Geometry: final body of the model. Coordinates: model frame, mm. A direction names the side the tool comes from. Coordinates: 2 decimals unless noted, no trailing zeros. Loops run counter-clockwise (first coordinate to the right, second up) from the corner with the lowest first, then second, coordinate; pieces in that order, holes last. Notation, with made-up numbers: (39.5, 24.5) - (72.5, 24.5) arc R24 ccw to (72.5, 51.5) - close; hole circle Ø1 at (53, -32.5). An arc over 180 degrees is marked (long way). Return JSON: item names as keys, results as strings.
from build123d import *

# Parameters (mm, degrees)
SKETCH1_R           = 4
SKETCH1_R_2         = 6
SKETCH1_R_3         = 9
BOSS_EXTRUDE1_DEPTH = 8
SKETCH2_R           = 4
BOSS_EXTRUDE2_DEPTH = 3
SKETCH3_R           = 6
BOSS_EXTRUDE3_DEPTH = 3


with BuildPart() as part:
    # Sketch1 → Boss-Extrude1 (new body)
    with BuildSketch(Plane(origin=(0, 0, 0), x_dir=(1, 0, 0), z_dir=(0, 1, 0))):
        with BuildLine():
            Line((82, 0), (0, 0))
            Line((0, 0), (-45.003147253, 18.182451735))
            ThreePointArc((-45.003147253, 18.182451735), (-54.304086029, 15.690272701), (-54.472135955, 6.06269888))
            Line((-54.472135955, 6.06269888), (-18.061799059, -44.051830542))
            ThreePointArc((-18.061799059, -44.051830542), (-9.061799059, -50.590713294), (2.062812738, -50.590713294))
            Line((2.062812738, -50.590713294), (85.708203932, -23.412678196))
            ThreePointArc((85.708203932, -23.412678196), (93.852260087, -10.12278642), (82, 0))
        make_face()
        with Locations(Location((-48, 10.764980899, 0), (0, 0, 270))):
            Circle(SKETCH1_R, mode=Mode.SUBTRACT)
        with Locations(Location((82, -12, 0), (0, 0, 270))):
            Circle(SKETCH1_R_2, mode=Mode.SUBTRACT)
        with Locations(Location((-3.49949316, -33.471696, 0), (0, 0, 270))):
            Circle(SKETCH1_R_3, mode=Mode.SUBTRACT)
    extrude(amount=BOSS_EXTRUDE1_DEPTH)

    # Sketch2 → Boss-Extrude2 (add, symmetric)
    with BuildSketch(Plane(origin=(-7.04036219, 0, -9.690227231), x_dir=(0.809016994374944, 0, -0.5877852522924779), z_dir=(0.5877852522924779, 0, 0.809016994374944))):
        with BuildLine():
            Line((-40.505318717, 8), (-40.505318717, 46))
            ThreePointArc((-40.505318717, 46), (-33.618703524, 53.92214455), (-24.815225149, 48.205098847))
            Line((-24.815225149, 48.205098847), (-13.286598571, 8))
            Line((-13.286598571, 8), (-40.505318717, 8))
        make_face()
        with Locations(Location((-32.505318717, 46, 0), (0, 0, 180))):
            Circle(SKETCH2_R, mode=Mode.SUBTRACT)
    extrude(amount=BOSS_EXTRUDE2_DEPTH, both=True)

    # Sketch3 → Boss-Extrude3 (add, symmetric)
    with BuildSketch(Plane(origin=(22.186685165, 0, -7.208891004), x_dir=(-0.30901699437494223, 0, -0.9510565162951553), z_dir=(0.9510565162951552, 0, -0.3090169943749422))):
        with BuildLine():
            Line((-48.752071734, 8), (-48.752071734, 48))
            ThreePointArc((-48.752071734, 48), (-38.006413293, 59.934262744), (-25.014300525, 50.49494029))
            Line((-25.014300525, 50.49494029), (-15.981722129, 8))
            Line((-15.981722129, 8), (-48.752071734, 8))
        make_face()
        with Locations((-36.752071734, 48)):
            Circle(SKETCH3_R, mode=Mode.SUBTRACT)
    extrude(amount=BOSS_EXTRUDE3_DEPTH, both=True)


solid = part.part
Item 1: Reachability of faces 4 (the face through (-9.21, 3.94, 50.54)), 5 (the face through (-29.33, 26.21, 10.21)), 6 (the face through (42, 4, 0)), 7 (the face through (36.1, 28.6, 25.9)) from +Z, -Z, +X, -X, +Y, -Y: full face, straight path, thin tool, end or side. Return the list, or none.
Worked out:
{"face 4": "+Z, +Y, -Y", "face 5": "+Z, +Y", "face 6": "-Z, +X, +Y, -Y", "face 7": "-Z, +X, +Y"}
Item 2: First-contact query: pin 1 Ø6.5 at (x, y) = (39, 6) entering from -Z; pin 2 Ø6 at (y, z) = (14.5, 32) entering from -X; pin 3 Ø1 at (y, z) = (9.5, 25) entering from -X. Flat tips, straight axial feed; report the tip coordinate or a pass-through.
Worked out:
{"pin 1": "z = 0", "pin 2": "x = 30.8", "pin 3": "x = 29.34"}
Item 3: Mould query, pull axis X, two halves, no side actions, for faces 1 (the face through (18, 0, 16)), 2 (the face through (34.047, 59.906, 29.157)), 3 (the face through (-32.941, 42.034, 9.076)). Classes: +X half, -X half, draft (parallel to the pull), parting line (faces both ways), or undercut.
Worked out:
{"face 1": "draft", "face 2": "parting line", "face 3": "undercut"}
Item 4: Section query C-C, the plane x = -23.5. Return loops of the section in (y, z), and give its area (3 significant figures).
Worked out:
{"outline": "(0, -9.49) - (8, -9.49) - (8, -1.44) - (25.02, -1.44) - (40.22, 5.98) - (8, 5.98) - (8, 36.57) - (0, 36.57) - close", "area": "551 mm^2"}
Item 5: Section query B-B, the plane x = -48. Return loops of the section in (y, z), and give its area (3 significant figures).
Worked out:
{"outline": "(0, -18.76) - (8, -18.76) - (8, -14.76) - (0, -14.76) - close; (0, -6.76) - (8, -6.76) - (8, 2.85) - (0, 2.85) - close", "area": "109 mm^2"}
Item 6: Section query A-A, the plane y = 16. Return loops of the section in (x, z), and give its area (3 significant figures).
Worked out:
{"outline": "(-41.57, 11.69) - (-21.41, -2.96) - (-17.88, 1.89) - (-38.05, 16.55) - close; (24.8, 10.53) - (30.5, 8.68) - (40.11, 38.23) - (34.4, 40.08) - close", "area": "336 mm^2"}
Item 7: Ray query, probe 1 along Y at (x, z) = (29.5, 31); probe 2 along X at (y, z) = (6.5, 14); probe 3 along X at (y, z) = (7.5, -11.5). Return the intervals inside material, ascending. Write a range as from..to.
Worked out:
{"probe 1": "0..8", "probe 2": "-39.9..76.34, 87.66..93.83", "probe 3": "-55.97..-51.93, -44.07..-28.46"}
Item 8: Section query D-D, the plane x = 8.5. Return loops of the section in (y, z), and give its area (3 significant figures).
Worked out:
{"outline": "(0, 0) - (8, 0) - (8, 48.5) - (0, 48.5) - close", "area": "388 mm^2"}
